The listing builds one solid part. Answer for the finished solid, in the listing's coordinates (mm). Face numbers are marked on the shaded views. A direction names the side the tool comes from. Coordinates: 2 decimals unless noted, no trailing zeros. Order: outer loops, then holes, each group sorted by start corner. A loop starts at its lowest first (then second) coordinate and runs counter-clockwise, first axis right, second up. Notation, with made-up numbers: (-35.5, -26) - (-1.5, -26) arc R33 cw to (-1.5, 5) - close; hole circle Ø10 at (31.5, 56.5). An arc over 180 degrees is marked (long way). Use one line per item in the form item = value. Start each with the question number.
Item 1: Section B-B, the plane z = -93 is taken. Write down the section's boundary in (x, y).
Item 2: Consider line 1 along Y through (x, z) = (0.5, -35); line 2 along Y through (x, z) = (-58.5, -136); line 3 along Z through (x, y) = (-96, 2.75). Determine where each line is inside the solid, lowest interval first. Write a range as [from, to].
Item 3: Section C-C, the plane x = -159 is taken. Write down the section's boundary in (y, z).
Item 4: Section A-A, the plane y = 15.5 is taken. Write down the section's boundary in (x, z).
Item 5: Each of these flat-tipped pins is pushed along its axis until it touches: pin 1 Ø2.5 at (x, y) = (-136.5, 5) entering from +Z; pin 2 Ø3 at (x, y) = (-220.5, 17) entering from +Z; pin 3 Ø1 at (x, y) = (-168, 9) entering from +Z; pin 4 Ø6 at (x, y) = (-77.5, 14) entering from +Z. Where does it stop, or does it pass through?
Item 6: Section D-D, the plane y = 5 is taken. Write down the section's boundary in (x, z), and give its area (3 significant figures).
Item 7: A tool of negligible diameter and unlimited length cuts with its end or side. For the marked faces 1, 2 and 3, from which of +Z, -Z, +X, -X, +Y, -Y can it reach the whole face along a straight path? Write none if from no direction.
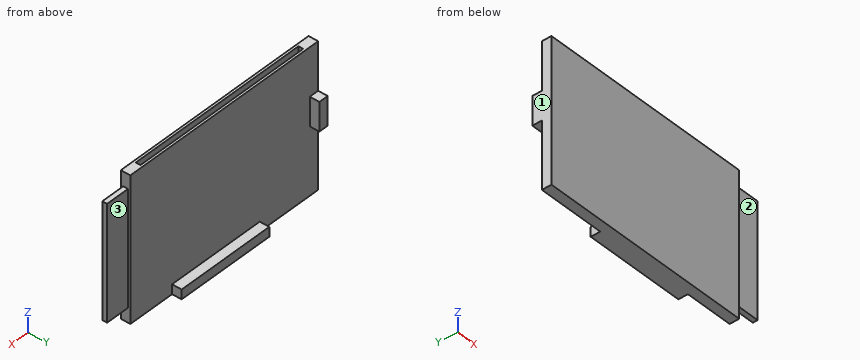
Autodesk Inventor part; units mm, degrees
ref_plane "YZ Plane" through (0, 0, 0) normal (1, 0, 0) x (0, 1, 0)
ref_plane "XZ Plane" through (0, 0, 0) normal (0, 1, 0) x (-1, 0, 0)
ref_plane "XY Plane" through (0, 0, 0) normal (0, 0, 1) x (1, 0, 0)
sketch "Sketch1" plane through (0, 0, 0) normal (0, 1, 0) x (-1, 0, 0)
  line L0 (0, 0) -> (225, 0)
  line L1 (225, 0) -> (225, -150)
  line L2 (225, -150) -> (0, -150)
  line L3 (0, -150) -> (0, 0)
  dimension "d0" = 225
  dimension "d1" = 150
extrude "Extrusion1" add sketch "Sketch1" along normal blind 10
sketch "Sketch2" plane through (0, 0, 0) normal (1, 0, 0) x (0, 0, -1)
  line L0 (0, 7.5) -> (150, 7.5)
  line L1 (150, 7.5) -> (150, 2.5)
  line L2 (150, 2.5) -> (0, 2.5)
  line L3 (0, 2.5) -> (0, 7.5)
  line L4 (150, 7.5) -> (135, 7.5)
  line L5 (135, 7.5) -> (135, 1.8795)
  line L6 (135, 1.8795) -> (150, 1.8795)
  line L7 (150, 1.8795) -> (150, 7.5)
  line L8 (0, 2.5) -> (15, 2.5)
  line L9 (15, 2.5) -> (15, 7.5)
  line L10 (15, 7.5) -> (0, 7.5)
  line L11 (0, 7.5) -> (0, 2.5)
  point P0 (0, 0)
  point P1 (135, 2.5)
  dimension "d4" = 150
  dimension "d5" = 5
  dimension "d6" = 15
  dimension "d7" = 15
sketch "Sketch3" plane through (-225, 0, 0) normal (0, 0, 1) x (1, 0, 0)
  line L0 (0, 7.5) -> (225, 7.5)
  line L1 (225, 7.5) -> (225, 2.5)
  line L2 (225, 2.5) -> (0, 2.5)
  line L3 (0, 2.5) -> (0, 7.5)
  line L4 (225, 7.5) -> (210, 7.5)
  line L5 (210, 7.5) -> (210, 2.5)
  line L6 (210, 2.5) -> (225, 2.5)
  line L7 (225, 2.5) -> (225, 7.5)
  line L8 (0, 7.5) -> (15, 7.5)
  line L9 (15, 7.5) -> (15, 2.5)
  line L10 (15, 2.5) -> (0, 2.5)
  line L11 (0, 2.5) -> (0, 7.5)
  point P0 (225, 0)
  dimension "d8" = 5
  dimension "d9" = 15
  dimension "d10" = 5
  dimension "d11" = 15
  dimension "d12" = 5
extrude "Extrusion2" cut sketch "Sketch3" against normal blind 25 contours L0 L5 L2 L9
extrude "Extrusion3" add sketch "Sketch2" along normal blind 25 contours L0 L5 L2 L9
sketch "Sketch4" plane through (0, 10, 0) normal (0, 1, 0) x (1, 0, 0)
  line L0 (-225, 150) -> (-225, 0)
  line L1 (-225, 50) -> (-215, 50)
  line L2 (-215, 50) -> (-215, 80)
  line L3 (-215, 80) -> (-225, 80)
  line L4 (-225, 80) -> (-225, 50)
  line L5 (0, 150) -> (-225, 150)
  line L6 (-50, 150) -> (-155, 150)
  line L7 (-155, 150) -> (-155, 140)
  line L8 (-155, 140) -> (-50, 140)
  line L9 (-50, 140) -> (-50, 150)
  point P0 (0, 0)
  dimension "d17" = 10
  dimension "d18" = 30
  dimension "d21" = 105
  dimension "d22" = 10
extrude "Extrusion4" add sketch "Sketch4" along normal blind 10
properties part number "TSU_FM_Floor"
Response:
q1.outline = (-225, 0) - (0, 0) - (0, 2.5) - (25, 2.5) - (25, 7.5) - (0, 7.5) - (0, 10) - (-225, 10) - close
q2.line_1 = [2.5, 7.5]
q2.line_2 = [0, 10]
q2.line_3 = [-150, -25]
q3.outline = (0, -150) - (10, -150) - (10, 0) - (7.5, 0) - (7.5, -25) - (2.5, -25) - (2.5, 0) - (0, 0) - close
q4.outline = (-225, -80) - (-215, -80) - (-215, -50) - (-225, -50) - close; (-155, -150) - (-50, -150) - (-50, -140) - (-155, -140) - close
q5.pin_1 = -25
q5.pin_2 = -50
q5.pin_3 = 0
q5.pin_4 = -140
q6.outline = (-225, -150) - (0, -150) - (0, -135) - (25, -135) - (25, -15) - (0, -15) - (0, 0) - (-15, 0) - (-15, -25) - (-210, -25) - (-210, 0) - (-225, 0) - close
q6.area = 31,900 mm2
q7.face_1 = +Z, -Z, -X, +Y, -Y
q7.face_2 = +Z, -Z, +X, -Y
q7.face_3 = +Z, -Z, +X, +Y
